Part model, mm, in its own coordinate system. A direction names the side the tool comes from. Give positions to 0.01 mm unless a question says otherwise; leave off trailing zeros. Answer as CSV lines item,"result". Start each with the question number.
Item 1: Wall check: L1, parallel to Y at x = 1, z = 1.5; L2, parallel to Y at x = -9.5, z = 1.5; L3, parallel to Y at x = -14.5, z = 0.5. Give the ranges that are in metal, low to high. Write a range as from..to.
Item 2: 3-axis set-ups, long thin cutter, end or side, ignore diameter. For faces 1 (the flat face through (-8.372, 14.384, 3.549)), 2 (the cylindrical face through (-1.97, 1.99, 3.45)), 3 (the flat face through (1, 1, 0)): which of +Z, -Z, +X, -X, +Y, -Y reach the whole face in a straight line?
Item 3: Pin check, flat tips, straight feed: pin 1 (2 mm diameter, centred on y = -11, z = 5, fed in from +X); pin 2 (3 mm diameter, centred on x = -11, z = 4.5, fed in from +Y); pin 3 (2 mm diameter, centred on x = 12, z = 3.5, fed in from +Y). Stop position of each tip, or through.
Item 4: Band-saw the part on A-A, the plane y = 6. Count the separate pieces of the cut face and the enclosed holes in it, then the cut area to 3 significant figures.
Item 5: Two-plate mould, pull along X, no slides. Class faces 4 (the flat face through (1, -1, 7)), 5 (the flat face through (8.372, -14.384, 3.549)): +X half, -X half, draft (parallel to the pull), parting line (faces both ways), or undercut.
from build123d import *

# Parameters (mm, degrees)
F0_W       = 35
F0_H       = 35
F2_W       = 28
F2_H       = 28
F4_T       = -1.2
F6_DEPTH   = 7
F7_SIZE2   = 3
F7_SIZE    = 6
F7_2_SIZE2 = 3
F7_2_SIZE  = 6
F7_3_SIZE2 = 3
F7_3_SIZE  = 6
F7_4_SIZE2 = 3
F7_4_SIZE  = 6


with BuildPart() as f3:
    # F0 (on Top) → F3 section 0
    with BuildSketch(Plane.XY):
        Rectangle(F0_W, F0_H)
    # F2 (on offset) → F3 section 1
    with BuildSketch(Plane.XY.offset(7)):
        Rectangle(F2_W, F2_H)
    loft()

    # F4
    f4_openings = [f3.faces().sort_by_distance(p)[0] for p in [
        (0, 0, 7),
        (0, 0, 0),
    ]]
    offset(amount=F4_T, openings=f4_openings)


with BuildPart() as f6:
    # F5 (on Top) → F6 (new body, through all)
    with BuildSketch(Plane.XY):
        with BuildLine():
            ThreePointArc((-2.683281573, -0.8), (-2.8, 0), (-2.683281573, 0.8))
            Line((-2.683281573, 0.8), (-16.2, 0.8))
            Line((-16.2, 0.8), (-16.2, -0.8))
            Line((-16.2, -0.8), (-2.683281573, -0.8))
        make_face()
        with BuildLine():
            ThreePointArc((-0.894427191, -0.8), (-1.2, 0), (-0.894427191, 0.8))
            Line((-0.894427191, 0.8), (-2.683281573, 0.8))
            ThreePointArc((-2.683281573, 0.8), (-2.8, 0), (-2.683281573, -0.8))
            Line((-2.683281573, -0.8), (-0.894427191, -0.8))
        make_face()
        with BuildLine():
            ThreePointArc((-0.894427191, 0.8), (-0.8485281374, 0.8485281374), (-0.8, 0.894427191))
            Line((-0.8, 0.894427191), (-0.8, 2.683281573))
            ThreePointArc((-0.8, 2.683281573), (-1.9798989873, 1.9798989873), (-2.683281573, 0.8))
            Line((-2.683281573, 0.8), (-0.894427191, 0.8))
        make_face()
        with BuildLine():
            ThreePointArc((-0.8, 0.894427191), (0, 1.2), (0.8, 0.894427191))
            Line((0.8, 0.894427191), (0.8, 2.683281573))
            ThreePointArc((0.8, 2.683281573), (0, 2.8), (-0.8, 2.683281573))
            Line((-0.8, 2.683281573), (-0.8, 0.894427191))
        make_face()
        with BuildLine():
            ThreePointArc((-0.8, 2.683281573), (0, 2.8), (0.8, 2.683281573))
            Line((0.8, 2.683281573), (0.8, 16.2))
            Line((0.8, 16.2), (-0.8, 16.2))
            Line((-0.8, 16.2), (-0.8, 2.683281573))
        make_face()
        with BuildLine():
            ThreePointArc((0.8, 0.894427191), (0.8485281374, 0.8485281374), (0.894427191, 0.8))
            Line((0.894427191, 0.8), (2.683281573, 0.8))
            ThreePointArc((2.683281573, 0.8), (1.9798989873, 1.9798989873), (0.8, 2.683281573))
            Line((0.8, 2.683281573), (0.8, 0.894427191))
        make_face()
        with BuildLine():
            ThreePointArc((0.894427191, 0.8), (1.1210068308, 0.4281865077), (1.2, 0))
            ThreePointArc((1.2, 0), (1.1210068308, -0.4281865077), (0.894427191, -0.8))
            Line((0.894427191, -0.8), (2.683281573, -0.8))
            ThreePointArc((2.683281573, -0.8), (2.7706667433, -0.40423483), (2.8, 0))
            ThreePointArc((2.8, 0), (2.7706667433, 0.40423483), (2.683281573, 0.8))
            Line((2.683281573, 0.8), (0.894427191, 0.8))
        make_face()
        with BuildLine():
            Line((16.2, 0.8), (2.683281573, 0.8))
            ThreePointArc((2.683281573, 0.8), (2.7706667433, 0.40423483), (2.8, 0))
            ThreePointArc((2.8, 0), (2.7706667433, -0.40423483), (2.683281573, -0.8))
            Line((2.683281573, -0.8), (16.2, -0.8))
            Line((16.2, -0.8), (16.2, 0.8))
        make_face()
        with BuildLine():
            Line((2.683281573, -0.8), (0.894427191, -0.8))
            ThreePointArc((0.894427191, -0.8), (0.8485281374, -0.8485281374), (0.8, -0.894427191))
            Line((0.8, -0.894427191), (0.8, -2.683281573))
            ThreePointArc((0.8, -2.683281573), (1.9798989873, -1.9798989873), (2.683281573, -0.8))
        make_face()
        with BuildLine():
            Line((-0.8, -2.683281573), (-0.8, -0.894427191))
            ThreePointArc((-0.8, -0.894427191), (-0.8485281374, -0.8485281374), (-0.894427191, -0.8))
            Line((-0.894427191, -0.8), (-2.683281573, -0.8))
            ThreePointArc((-2.683281573, -0.8), (-1.9798989873, -1.9798989873), (-0.8, -2.683281573))
        make_face()
        with BuildLine():
            Line((0.8, -2.683281573), (0.8, -0.894427191))
            ThreePointArc((0.8, -0.894427191), (0, -1.2), (-0.8, -0.894427191))
            Line((-0.8, -0.894427191), (-0.8, -2.683281573))
            ThreePointArc((-0.8, -2.683281573), (0, -2.8), (0.8, -2.683281573))
        make_face()
        with BuildLine():
            Line((0.8, -16.2), (0.8, -2.683281573))
            ThreePointArc((0.8, -2.683281573), (0, -2.8), (-0.8, -2.683281573))
            Line((-0.8, -2.683281573), (-0.8, -16.2))
            Line((-0.8, -16.2), (0.8, -16.2))
        make_face()
    extrude(amount=F6_DEPTH)

    # F7
    f7_edges = [f6.edges().sort_by_distance(p)[0] for p in [
        (-16.2, 0, 7),
    ]]
    f7_side = f6.faces().sort_by_distance((-16.2, 0, 3.5))[0]
    chamfer(f7_edges, length=F7_SIZE, length2=F7_SIZE2, reference=f7_side)

    # F7#2
    f7_2_edges = [f6.edges().sort_by_distance(p)[0] for p in [
        (0, 16.2, 7),
    ]]
    f7_2_side = f6.faces().sort_by_distance((0, 16.2, 3.5))[0]
    chamfer(f7_2_edges, length=F7_2_SIZE, length2=F7_2_SIZE2, reference=f7_2_side)

    # F7#3
    f7_3_edges = [f6.edges().sort_by_distance(p)[0] for p in [
        (16.2, 0, 7),
    ]]
    f7_3_side = f6.faces().sort_by_distance((16.2, 0, 3.5))[0]
    chamfer(f7_3_edges, length=F7_3_SIZE, length2=F7_3_SIZE2, reference=f7_3_side)

    # F7#4
    f7_4_edges = [f6.edges().sort_by_distance(p)[0] for p in [
        (0, -16.2, 7),
    ]]
    f7_4_side = f6.faces().sort_by_distance((0, -16.2, 3.5))[0]
    chamfer(f7_4_edges, length=F7_4_SIZE, length2=F7_4_SIZE2, reference=f7_4_side)


with BuildPart() as f3_1:
    add(f3.part)

    # F8: union F6
    add(f6.part)


solid = f3_1.part
Output:
1,L1,"-16.75..-15.41, -2.62..-0.66, 0.66..2.62, 15.41..16.75"
1,L2,"-16.75..-15.41, -0.8..0.8, 15.41..16.75"
1,L3,"-17.25..-15.91, -0.8..0.8, 15.91..17.25"
2,face 1,"-Z"
2,face 2,"+Z, -Z"
2,face 3,"-Z, +X, -X, +Y, -Y"
3,pin 1,"x = 15.5"
3,pin 2,"y = 16"
3,pin 3,"y = 16.25"
4,separate pieces,"3"
4,enclosed holes,"0"
4,area,"30.0 mm²"
5,face 4,"draft"
5,face 5,"undercut"
